```python
from build123d import *

# Parameters (mm, degrees)
SKETCH_1_R      = 10
EXTRUDE_3_DEPTH = 20


with BuildPart() as part:
    # Эскиз1 → Бобышка-Вытянуть3 (new body)
    with BuildSketch(Plane.XY):
        with BuildLine():
            Line((-15.578628424, 110.843660763), (-11.436492801, 114.985796387))
            ThreePointArc((-11.436492801, 114.985796387), (-8.192259312, 117.1535239), (-4.365424989, 117.914728575))
            Line((-4.365424989, 117.914728575), (-2.649696236, 117.914728575))
            ThreePointArc((-2.649696236, 117.914728575), (1.177138088, 117.1535239), (4.421371576, 114.985796387))
            Line((4.421371576, 114.985796387), (8.563507199, 110.843660763))
            ThreePointArc((8.563507199, 110.843660763), (10.731234713, 107.599427275), (11.492439388, 103.772592951))
            Line((11.492439388, 103.772592951), (11.492439388, 32.914728575))
            ThreePointArc((11.492439388, 32.914728575), (17.350303764, 18.772592951), (31.492439388, 12.914728575))
            Line((31.492439388, 12.914728575), (102.350303764, 12.914728575))
            ThreePointArc((102.350303764, 12.914728575), (106.177138088, 12.1535239), (109.421371576, 9.985796387))
            Line((109.421371576, 9.985796387), (113.563507199, 5.843660763))
            ThreePointArc((113.563507199, 5.843660763), (115.731234713, 2.599427275), (116.492439388, -1.227407049))
            Line((116.492439388, -1.227407049), (116.492439388, -2.943135801))
            ThreePointArc((116.492439388, -2.943135801), (115.731234713, -6.769970125), (113.563507199, -10.014203613))
            Line((113.563507199, -10.014203613), (109.421371576, -14.156339237))
            ThreePointArc((109.421371576, -14.156339237), (106.177138088, -16.32406675), (102.350303764, -17.085271425))
            Line((102.350303764, -17.085271425), (31.492439388, -17.085271425))
            ThreePointArc((31.492439388, -17.085271425), (17.350303764, -22.943135801), (11.492439388, -37.085271425))
            Line((11.492439388, -37.085271425), (11.492439388, -107.943135801))
            ThreePointArc((11.492439388, -107.943135801), (10.731234713, -111.769970125), (8.563507199, -115.014203613))
            Line((8.563507199, -115.014203613), (4.421371576, -119.156339237))
            ThreePointArc((4.421371576, -119.156339237), (1.177138088, -121.32406675), (-2.649696236, -122.085271425))
            Line((-2.649696236, -122.085271425), (-4.365424989, -122.085271425))
            ThreePointArc((-4.365424989, -122.085271425), (-8.192259312, -121.32406675), (-11.436492801, -119.156339237))
            Line((-11.436492801, -119.156339237), (-15.578628424, -115.014203613))
            ThreePointArc((-15.578628424, -115.014203613), (-17.746355937, -111.769970125), (-18.507560612, -107.943135801))
            Line((-18.507560612, -107.943135801), (-18.507560612, -37.085271425))
            ThreePointArc((-18.507560612, -37.085271425), (-24.365424989, -22.943135801), (-38.507560612, -17.085271425))
            Line((-38.507560612, -17.085271425), (-109.365424989, -17.085271425))
            ThreePointArc((-109.365424989, -17.085271425), (-113.192259312, -16.32406675), (-116.436492801, -14.156339237))
            Line((-116.436492801, -14.156339237), (-120.578628424, -10.014203613))
            ThreePointArc((-120.578628424, -10.014203613), (-122.746355937, -6.769970125), (-123.507560612, -2.943135801))
            Line((-123.507560612, -2.943135801), (-123.507560612, -1.227407049))
            ThreePointArc((-123.507560612, -1.227407049), (-122.746355937, 2.599427275), (-120.578628424, 5.843660763))
            Line((-120.578628424, 5.843660763), (-116.436492801, 9.985796387))
            ThreePointArc((-116.436492801, 9.985796387), (-113.192259312, 12.1535239), (-109.365424989, 12.914728575))
            Line((-109.365424989, 12.914728575), (-38.507560612, 12.914728575))
            ThreePointArc((-38.507560612, 12.914728575), (-24.365424989, 18.772592951), (-18.507560612, 32.914728575))
            Line((-18.507560612, 32.914728575), (-18.507560612, 103.772592951))
            ThreePointArc((-18.507560612, 103.772592951), (-17.746355937, 107.599427275), (-15.578628424, 110.843660763))
        make_face()
        with Locations((-103.507560612, -2.085271425)):
            Circle(SKETCH_1_R, mode=Mode.SUBTRACT)
        with Locations((-3.507560612, 97.914728575)):
            Circle(SKETCH_1_R, mode=Mode.SUBTRACT)
        with Locations((96.492439388, -2.085271425)):
            Circle(SKETCH_1_R, mode=Mode.SUBTRACT)
        with Locations((-3.507560612, -102.085271425)):
            Circle(SKETCH_1_R, mode=Mode.SUBTRACT)
    extrude(amount=EXTRUDE_3_DEPTH)


solid = part.part
```
Model file for the job. Use its own axes, mm. A direction names the side the tool comes from. Coordinates: 2 decimals unless noted, no trailing zeros. Write each loop counter-clockwise with the first axis right and the second up, starting at its lowest first coordinate (ties: lowest second). Pieces come first, ordered by that corner, then holes. Notation, with made-up numbers: (30.5, 54) - (72.5, 54) arc R21 ccw to (72.5, 85) - close; hole circle Ø8 at (15.5, 61.25). An arc over 180 degrees is marked (long way). Use a Markdown table: item, result. Add a question column.
Item 1: Band-saw the part on A-A, the plane x = -103.5. Write the cut outline in (y, z).
Item 2: Band-saw the part on B-B, the plane y = -7. Write the cut outline in (x, z).
Item 3: Drill centre lines: line 1 along X through (y, z) = (6, 3.75); line 2 along Y through (x, z) = (97.5, 14); line 3 along X through (y, z) = (-6.5, 15.75). Where is each one in solid material? Low to high.
Item 4: Drop flat-ended pins along their axis: pin 1 (6 mm diameter, centred on y = 34.5, z = 4.5, fed in from +X); pin 2 (10 mm diameter, centred on y = 26.5, z = 15.5, fed in from +X); pin 3 (6 mm diameter, centred on y = -55.5, z = 13, fed in from -X). Give the stop position or say it passes through.
Item 5: Band-saw the part on D-D, the plane x = 65. Write the cut outline in (y, z).
Item 6: 3-axis set-ups, long thin cutter, end or side, ignore diameter. For faces 5 (the face through (-18.508, 68, 10)), 6 (the face through (-18.508, -73, 10)), 7 (the face through (67, -17.085, 10)), 8 (the face through (-113.5, -1.65, 9.86)): which of +Z, -Z, +X, -X, +Y, -Y reach the whole face in a straight line?
Item 7: Two-plate mould, pull along X, no slides. Class faces 1 (the face through (-17.725, -111.821, 9.86)), 2 (the face through (-3, -2, 0)), 3 (the face through (1.868, 106.347, 9.86)), 4 (the face through (1.23, -121.3, 9.86)): pulls with the +X half, pulls with the -X half, needs draft (parallel to the pull), parting line crosses it, or undercut.
Item 8: Band-saw the part on C-C, the plane y = 91. Write the cut outline in (x, z), and give its area (3 significant figures).
A:
| question | item | result |
|---|---|---|
| 1 | outline | (-17.09, 0) - (-12.09, 0) - (-12.09, 20) - (-17.09, 20) - close; (7.91, 0) - (12.91, 0) - (12.91, 20) - (7.91, 20) - close |
| 2 | outline | (-122.65, 0) - (-112.22, 0) - (-112.22, 20) - (-122.65, 20) - close; (-94.8, 0) - (87.78, 0) - (87.78, 20) - (-94.8, 20) - close; (105.2, 0) - (115.63, 0) - (115.63, 20) - (105.2, 20) - close |
| 3 | line 1 | x = -120.42 to -109.39, -97.62 to 90.61, 102.38 to 113.41 |
| 3 | line 2 | y = -17.09 to -12.03, 7.86 to 12.91 |
| 3 | line 3 | x = -122.85 to -112.48, -94.53 to 87.52, 105.47 to 115.84 |
| 4 | pin 1 | stops at x = 11.54 |
| 4 | pin 2 | stops at x = 15.07 |
| 4 | pin 3 | stops at x = -18.51 |
| 5 | outline | (-17.09, 0) - (12.91, 0) - (12.91, 20) - (-17.09, 20) - close |
| 6 | face 5 | +Z, -Z, -X, +Y |
| 6 | face 6 | +Z, -Z, -X, -Y |
| 6 | face 7 | +Z, -Z, +X, -Y |
| 6 | face 8 | +Z, -Z |
| 7 | face 1 | pulls with the -X half |
| 7 | face 2 | needs draft |
| 7 | face 3 | undercut |
| 7 | face 4 | pulls with the +X half |
| 8 | outline | (-18.51, 0) - (-10.73, 0) - (-10.73, 20) - (-18.51, 20) - close; (3.72, 0) - (11.49, 0) - (11.49, 20) - (3.72, 20) - close |
| 8 | area | 311 mm² |
